Model file for the job. Use its own axes, mm. A direction names the side the tool comes from. Give positions to 0.01 mm unless a question says otherwise; leave off trailing zeros. Write each loop counter-clockwise with the first axis right and the second up, starting at its lowest first coordinate (ties: lowest second). Pieces come first, ordered by that corner, then holes. Notation, with made-up numbers: (-0.5, 39) - (50.5, 39) arc R20 cw to (50.5, 63) - close; hole circle Ø7 at (-8, 35). An arc over 180 degrees is marked (long way). One line per item, written item: value. Start each with the question number.
(1) Drop flat-ended pins along their axis: P1, Ø1.8, axis at x = -12, y = -43.5, coming from the +Z side; P2, Ø4.5, axis at x = -13.5, z = 57, coming from the -Y side; P3, Ø1, axis at x = -5, y = 18.5, coming from the -Z side; P4, Ø6, axis at x = 11.5, z = 56, coming from the +Y side. Give the stop position or say it passes through.
(2) Mould opens along Z. For faces 1 (the face through (0, -12.5, -3)), 2 (the face through (-11, 39, 10)), 3 (the face through (0.1, 30.4, 90)) say: pulls with the +Z half, pulls with the -Z half, needs draft (parallel to the pull), parting line crosses it, or undercut.
(3) 3-axis set-ups, long thin cutter, end or side, ignore diameter. For faces 4 (the face through (13, 40, -8)), 5 (the face through (11, -40, 10)), 6 (the face through (13, -39, -8)): which of +Z, -Z, +X, -X, +Y, -Y reach the whole face in a straight line?
(4) Cut at C-C, the plane z = 106. List the corners of the cut face in (x, y).
(5) Cut at D-D, the plane y = -10. List the corners of the cut face in (x, z), and give its area (3 significant figures).
(6) Cut at B-B, the plane z = 43. List the corners of the cut face in (x, y).
(7) Probe L1, parallel to Y at x = 6.75, z = 80; L2, parallel to Z at x = -4.25, y = 11; L3, parallel to X at y = -16, z = -3.5. List the from-to ranges inside material, lowest first.
(8) Cut at A-A, the plane x = -11.5. List the corners of the cut face in (y, z), and give its area (3 significant figures).
from build123d import *

# Parameters (mm, degrees)
SKETCH1_W           = 30
SKETCH1_H           = 25
BOSS_EXTRUDE1_DEPTH = 115
BOSS_EXTRUDE2_DEPTH = 9.5
SKETCH4_W           = 11.5
SKETCH4_H           = 6.5
CUT_EXTRUDE1_DEPTH  = 151.552316488
BOSS_EXTRUDE3_DEPTH = 13
CUT_EXTRUDE2_DEPTH  = 128.000984248
FILLET1_R           = 2.5
FILLET2_R           = 2.5


with BuildPart() as part:
    # Sketch1 → Boss-Extrude1 (new body)
    with BuildSketch(Plane.XY):
        Rectangle(SKETCH1_W, SKETCH1_H)
    extrude(amount=BOSS_EXTRUDE1_DEPTH)

    # Sketch3 → Boss-Extrude2 (add, symmetric)
    with BuildSketch(Plane(origin=(0, 0, 0), x_dir=(0, 0, -1), z_dir=(1, 0, 0))):
        Polygon((5, -12.5), (0, -12.5), (-115, -12.5), (-115, -48), (25, -48), (25, -38), align=None)
        Polygon((-115, 48), (25, 48), (25, 38), (5, 12.5), (0, 12.5), (-115, 12.5), align=None)
    extrude(amount=BOSS_EXTRUDE2_DEPTH, both=True)

    # Sketch4 → Cut-Extrude1 (cut, through all)
    with BuildSketch(Plane(origin=(0, 48, 0), x_dir=(1, 0, 0), z_dir=(0, 1, 0))):
        with Locations((9.25, -111.75)):
            Rectangle(SKETCH4_W, SKETCH4_H)
    extrude(amount=-CUT_EXTRUDE1_DEPTH, mode=Mode.SUBTRACT)

    # Sketch6 → Boss-Extrude3 (add, symmetric)
    with BuildSketch(Plane(origin=(0, 0, 0), x_dir=(0, 0, -1), z_dir=(1, 0, 0))):
        Polygon((-10, 48), (25, 48), (25, 38), (19.509803922, 31), (-10, 31), align=None)
        Polygon((25, -48), (-10, -48), (-10, -31), (19.509803922, -31), (25, -38), align=None)
    extrude(amount=BOSS_EXTRUDE3_DEPTH, both=True)

    # Sketch7 → Cut-Extrude2 (cut, through all)
    with BuildSketch(Plane(origin=(9.5, 0, 0), x_dir=(0, 0, -1), z_dir=(1, 0, 0))):
        with BuildLine():
            Line((-84.5, 36), (-33.5, 36))
            ThreePointArc((-33.5, 36), (-28, 30.5), (-33.5, 25))
            Line((-33.5, 25), (-84.5, 25))
            ThreePointArc((-84.5, 25), (-90, 30.5), (-84.5, 36))
        make_face()
        with BuildLine():
            Line((-84.5, -27.384190741), (-33.5, -27.384190741))
            ThreePointArc((-33.5, -27.384190741), (-28, -32.884190741), (-33.5, -38.384190741))
            Line((-33.5, -38.384190741), (-84.5, -38.384190741))
            ThreePointArc((-84.5, -38.384190741), (-90, -32.884190741), (-84.5, -27.384190741))
        make_face()
    extrude(amount=-CUT_EXTRUDE2_DEPTH, mode=Mode.SUBTRACT)

    # Fillet1
    fillet1_edges = [part.edges().sort_by_distance(p)[0] for p in [
        (9.5, 30.5, 90),
        (9.5, 25, 59),
        (9.5, 30.5, 28),
        (9.5, 36, 59),
    ]]
    fillet(fillet1_edges, radius=FILLET1_R)

    # Fillet2
    fillet2_edges = [part.edges().sort_by_distance(p)[0] for p in [
        (-9.5, 25, 59),
        (-9.5, 30.5, 28),
        (-9.5, 36, 59),
        (-9.5, 30.5, 90),
        (-9.5, -38.384190741, 59),
        (-9.5, -32.884190741, 28),
        (-9.5, -27.384190741, 59),
        (-9.5, -32.884190741, 90),
        (9.5, -32.884190741, 90),
        (9.5, -38.384190741, 59),
        (9.5, -32.884190741, 28),
        (9.5, -27.384190741, 59),
    ]]
    fillet(fillet2_edges, radius=FILLET2_R)


solid = part.part
Answers follow:
1. P1: stops at z = 10
1. P2: stops at y = -12.5
1. P3: stops at z = -10.1
1. P4: stops at y = 48
2. face 1: needs draft
2. face 2: pulls with the +Z half
2. face 3: undercut
3. face 4: +Z, -Z, +X, +Y
3. face 5: +Z, +X, -Y
3. face 6: +Z, -Z, +X, -Y
4. outline: (-15, -12.5) - (-9.5, -12.5) - (-9.5, -48) - (9.5, -48) - (9.5, -12.5) - (15, -12.5) - (15, 12.5) - (9.5, 12.5) - (9.5, 48) - (-9.5, 48) - (-9.5, 12.5) - (-15, 12.5) - close
5. outline: (-15, 0) - (15, 0) - (15, 108.5) - (3.5, 108.5) - (3.5, 115) - (-15, 115) - close
5. area: 3,380 mm²
6. outline: (-15, -12.5) - (-9.5, -12.5) - (-9.5, -24.88) arc R2.5 ccw to (-7, -27.38) - (7, -27.38) arc R2.5 ccw to (9.5, -24.88) - (9.5, -12.5) - (15, -12.5) - (15, 12.5) - (9.5, 12.5) - (9.5, 22.5) arc R2.5 ccw to (7, 25) - (-7, 25) arc R2.5 ccw to (-9.5, 22.5) - (-9.5, 12.5) - (-15, 12.5) - close; (-9.5, -48) - (9.5, -48) - (9.5, -40.88) arc R2.5 ccw to (7, -38.38) - (-7, -38.38) arc R2.5 ccw to (-9.5, -40.88) - close; (-9.5, 38.5) arc R2.5 ccw to (-7, 36) - (7, 36) arc R2.5 ccw to (9.5, 38.5) - (9.5, 48) - (-9.5, 48) - close
7. L1: y = -48 to -38.38, -27.38 to 25, 36 to 48
7. L2: z = 0 to 115
7. L3: x = -9.5 to 9.5
8. outline: (-48, -25) - (-38, -25) - (-31, -19.51) - (-31, 10) - (-48, 10) - close; (-12.5, 0) - (12.5, 0) - (12.5, 115) - (-12.5, 115) - close; (31, -19.51) - (38, -25) - (48, -25) - (48, 10) - (31, 10) - close
8. area: 4,030 mm²
